The figure shows three views and two pictorial views of one solid part (mm, origin at its lowest corner). Answer the questions. A direction names the side the tool comes from. Round coordinates to 2 decimals unless told otherwise and drop trailing zeros. Write each loop counter-clockwise with the first axis right and the second up, starting at its lowest first coordinate (ties: lowest second). Pieces come first, ordered by that corner, then holes. Notation, with made-up numbers: M 16,1.5 L 52,1.5 A23 ccw 52,19.5 Z; hole C 9,78.5 d10. An arc over 180 degrees is marked long. Answer in a Markdown table with one row per item.
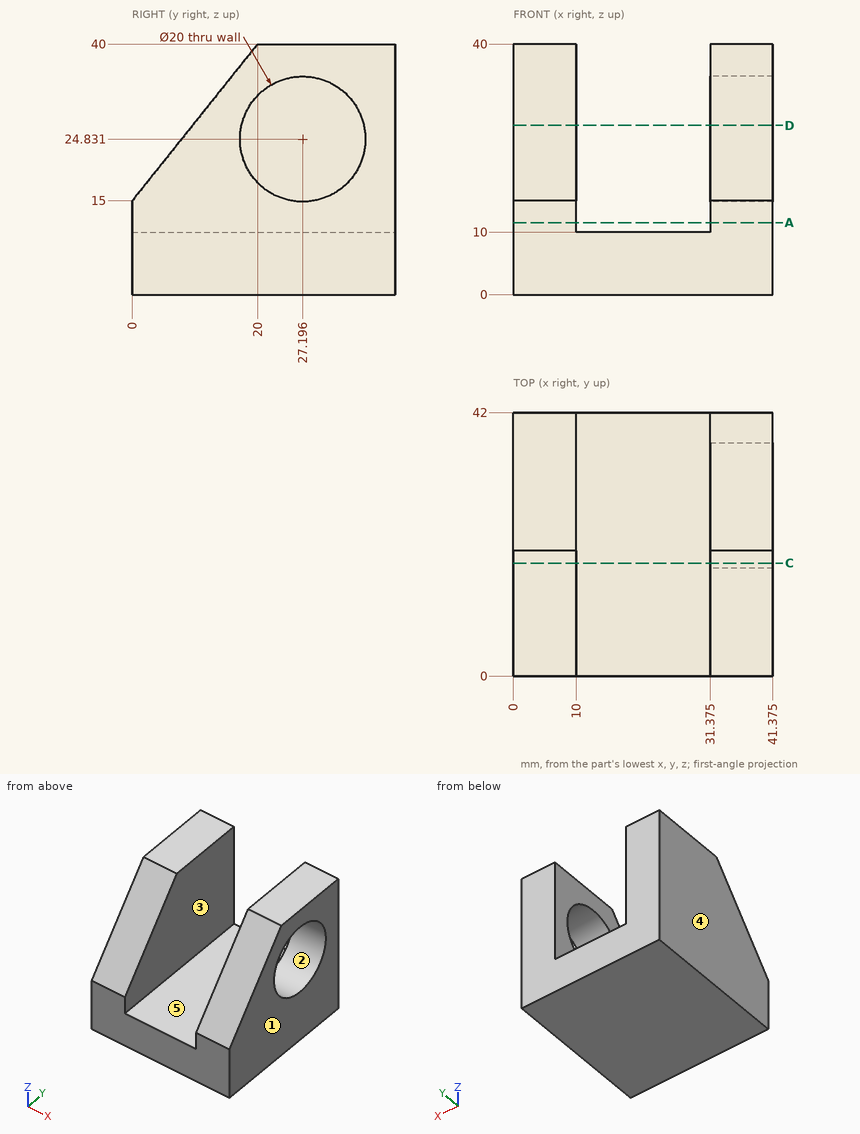
1. A tool of negligible diameter and unlimited length cuts with its end or side. For the marked faces 4 and 5, from which of +Z, -Z, +X, -X, +Y, -Y can it reach the whole face along a straight path? Write none if from no direction.
Calculated:
| item | result |
|---|---|
| face 4 | +Z, -Z, -X, +Y, -Y |
| face 5 | +Z, +Y, -Y |
2. Consider line 1 along X through (y, z) = (35.5, 11.5) (1 decimal); line 2 along Z through (x, y) = (38, 21.5); line 3 along Z through (x, y) = (13, 11). Determine where each line is inside the solid, lowest interval first. Write a range as from..to.
Calculated:
| item | result |
|---|---|
| line 1 | x = 0..10, 31.4..41.4 |
| line 2 | z = 0..16.61, 33.05..40 |
| line 3 | z = 0..10 |
3. Determine the mould class of the marked faces 1, 2 and 3 for opening direction X: released by +X, released by -X, zero draft, split by the parting line, or undercut.
Calculated:
| item | result |
|---|---|
| face 1 | released by +X |
| face 2 | zero draft |
| face 3 | undercut |
4. The part is cut by section A-A (z = 11.5). Determine the outline of the cut face in (x, y) (1 decimal), plus the area to 3 significant figures.
Calculated:
| item | result |
|---|---|
| outline | M 0,0 L 10,0 L 10,42 L 0,42 Z; M 31.4,0 L 41.4,0 L 41.4,42 L 31.4,42 Z |
| area | 840 mm² |
5. The part is cut by section D-D (z = 27). Determine the outline of the cut face in (x, y) (1 decimal).
Calculated:
| item | result |
|---|---|
| outline | M 0,9.6 L 10,9.6 L 10,42 L 0,42 Z; M 31.4,9.6 L 41.4,9.6 L 41.4,17.4 L 31.4,17.4 Z; M 31.4,37 L 41.4,37 L 41.4,42 L 31.4,42 Z |
6. Given pin 1 (3 mm diameter, centred on x = 6.5, y = 7, fed in from +Z) (1 decimal); pin 2 (10.5 mm diameter, centred on x = 23, y = 23, fed in from +Z); pin 3 (8 mm diameter, centred on x = 36, y = 6, fed in from +Z), each flat-ended and moving along its own axis, determine where each tip first touches the part or whether it passes through.
Calculated:
| item | result |
|---|---|
| pin 1 | stops at z = 25.6 |
| pin 2 | stops at z = 10 |
| pin 3 | stops at z = 27.5 |
7. The part is cut by section C-C (y = 18). Determine the outline of the cut face in (x, z) (1 decimal), plus the area to 3 significant figures.
Calculated:
| item | result |
|---|---|
| outline | M 0,0 L 41.4,0 L 41.4,20.9 L 31.4,20.9 L 31.4,10 L 10,10 L 10,37.5 L 0,37.5 Z; M 31.4,28.8 L 41.4,28.8 L 41.4,37.5 L 31.4,37.5 Z |
| area | 885 mm² |
